from build123d import *

# Parameters (mm, degrees)
SKETCH_W        = 37.5
SKETCH_H        = 36
PAD_DEPTH       = 3.5
SKETCH001_R     = 1.05
POCKET_DEPTH    = 5
SKETCH002_R     = 1.6
POCKET001_DEPTH = 1.1
SKETCH003_W     = 10
SKETCH003_H     = 2.5
PAD001_DEPTH    = 5
SKETCH004_W     = 20
SKETCH004_H     = 2.5
PAD002_DEPTH    = 5
SKETCH005_W     = 7
SKETCH005_H     = 7
POCKET002_DEPTH = 5
FILLET_R        = 3
FILLET001_R     = 2


with BuildPart() as part:
    # Sketch → Pad (new body)
    with BuildSketch(Plane.XY):
        Rectangle(SKETCH_W, SKETCH_H)
    extrude(amount=PAD_DEPTH)

    # Sketch001 (on Face6 of Pad) → Pocket (cut)
    with BuildSketch(Plane.XY.offset(3.5)):
        with Locations((0, -14.25)):
            Circle(SKETCH001_R)
    extrude(amount=-POCKET_DEPTH, mode=Mode.SUBTRACT)

    # Sketch002 (on Face5 of Pocket) → Pocket001 (cut)
    with BuildSketch(Plane.XY.offset(3.5)):
        with Locations((0, -14.25)):
            Circle(SKETCH002_R)
    extrude(amount=-POCKET001_DEPTH, mode=Mode.SUBTRACT)

    # Sketch003 (on Face4 of Pocket001) → Pad001 (join)
    with BuildSketch(Plane(origin=(0, 0, 0), x_dir=(1, 0, 0), z_dir=(0, 0, -1))):
        with Locations((-10, 14.6)):
            Rectangle(SKETCH003_W, SKETCH003_H)
        with Locations((10, 14.6)):
            Rectangle(SKETCH003_W, SKETCH003_H)
    extrude(amount=PAD001_DEPTH)

    # Sketch004 (on Face4 of Pad001) → Pad002 (join)
    with BuildSketch(Plane(origin=(0, 0, 0), x_dir=(1, 0, 0), z_dir=(0, 0, -1))):
        with Locations((-4.75, -14.6)):
            Rectangle(SKETCH004_W, SKETCH004_H)
    extrude(amount=PAD002_DEPTH)

    # Sketch005 (on Face4 of Pad002) → Pocket002 (cut)
    with BuildSketch(Plane(origin=(0, 0, 0), x_dir=(1, 0, 0), z_dir=(0, 0, -1))):
        with Locations((15.25, -14.5)):
            Rectangle(SKETCH005_W, SKETCH005_H)
    extrude(amount=-POCKET002_DEPTH, mode=Mode.SUBTRACT)

    # Fillet
    fillet_edges = [part.edges().sort_by_distance(p)[0] for p in [
        (11.75, 11, 1.75),
    ]]
    fillet(fillet_edges, radius=FILLET_R)

    # Fillet001
    fillet001_edges = [part.edges().sort_by_distance(p)[0] for p in [
        (18.75, -18, 1.75),
        (-18.75, 18, 1.75),
        (-18.75, -18, 1.75),
    ]]
    fillet(fillet001_edges, radius=FILLET001_R)


solid = part.part
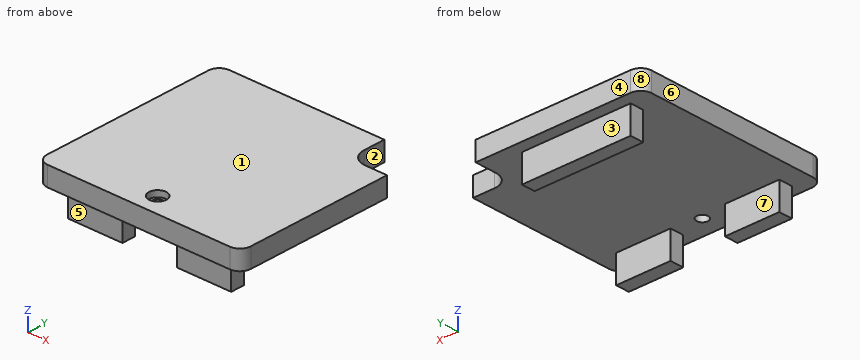
Verification items for the finished model (mm, model axes). Face numbers are marked on the shaded views. A direction names the side the tool comes from. Coordinates: 2 decimals unless noted, no trailing zeros. Order: outer loops, then holes, each group sorted by start corner. A loop starts at its lowest first (then second) coordinate and runs counter-clockwise, first axis right, second up. Notation, with made-up numbers: (11, 44.5) -> (33, 44.5) arc R20 ccw to (33, 48.5) -> close; hole circle Ø3 at (53.25, 31.25). An arc over 180 degrees is marked (long way). Put each result on its own line as item: value. Start each with the question number.
1. Cross-section at D-D, the plane z = 1.5. Record the boundary of the cut face in (x, y), then the cut area to 3 significant figures.
2. Cross-section at A-A, the plane x = 0. Record the boundary of the cut face in (y, z), then the cut area to 3 significant figures.
3. Mould release check, pull along Y, two halves, no side actions. Record for the marked faces 6, 7 and 8: released by +Y, released by -Y, zero draft, split by the parting line, or undercut.
4. Cross-section at C-C, the plane y = -14.25. Record the boundary of the cut face in (x, z), then the cut area to 3 significant figures.
5. Cross-section at B-B, the plane z = -3.75. Record the boundary of the cut face in (x, y).
6. Access from +Z, -Z, +X, -X, +Y, -Y to the whole of each face (thin tool, end or side, straight path). Record for the marked faces 1, 2, 3, 4 and 5.
7. Go/stop test with flat-tipped pins: pin 1 Ø1.2 at (y, z) = (14.5, -3.5) entering from -X; pin 2 Ø0.8 at (y, z) = (-15, -3) entering from +X; pin 3 Ø1 at (x, y) = (0, -14) entering from +Z; pin 4 Ø0.8 at (y, z) = (-15, -3.5) entering from -X. Record where each tip stops, or that it passes through.
8. Material ranges on L1, parallel to Y at x = -8, z = -4.25; L2, parallel to Y at x = 0, z = 3; L3, parallel to Z at x = 7.5, y = -3.5, recorded low to high. Write a range as [from, to].
Computed:
1. outline: (-18.75, -16) arc R2 ccw to (-16.75, -18) -> (16.75, -18) arc R2 ccw to (18.75, -16) -> (18.75, 11) -> (14.75, 11) arc R3 cw to (11.75, 14) -> (11.75, 18) -> (-16.75, 18) arc R2 ccw to (-18.75, 16) -> close; hole circle Ø2.1 at (0, -14.25)
1. area: 1,300 mm2
2. outline: (-18, 0) -> (-15.3, 0) -> (-15.3, 2.4) -> (-15.85, 2.4) -> (-15.85, 3.5) -> (-18, 3.5) -> close; (-13.2, 0) -> (13.35, 0) -> (13.35, -5) -> (15.85, -5) -> (15.85, 0) -> (18, 0) -> (18, 3.5) -> (-12.65, 3.5) -> (-12.65, 2.4) -> (-13.2, 2.4) -> close
2. area: 130 mm2
3. face 6: zero draft
3. face 7: undercut
3. face 8: released by +Y
4. outline: (-18.75, 0) -> (-15, 0) -> (-15, -5) -> (-5, -5) -> (-5, 0) -> (-1.05, 0) -> (-1.05, 2.4) -> (-1.6, 2.4) -> (-1.6, 3.5) -> (-18.75, 3.5) -> close; (1.05, 0) -> (5, 0) -> (5, -5) -> (15, -5) -> (15, 0) -> (18.75, 0) -> (18.75, 3.5) -> (1.6, 3.5) -> (1.6, 2.4) -> (1.05, 2.4) -> close
4. area: 223 mm2
5. outline: (-15, -15.85) -> (-5, -15.85) -> (-5, -13.35) -> (-15, -13.35) -> close; (-14.75, 13.35) -> (5.25, 13.35) -> (5.25, 15.85) -> (-14.75, 15.85) -> close; (5, -15.85) -> (15, -15.85) -> (15, -13.35) -> (5, -13.35) -> close
6. face 1: +Z, +X, -X, +Y, -Y
6. face 2: +Z, -Z, +X, +Y
6. face 3: -Z, +X, -X, +Y
6. face 4: +Z, -Z, +X, -X, +Y
6. face 5: -Z, +X, -X, -Y
7. pin 1: x = -14.75
7. pin 2: x = 15
7. pin 3: through
7. pin 4: x = -15
8. L1: [-15.85, -13.35], [13.35, 15.85]
8. L2: [-18, -15.85], [-12.65, 18]
8. L3: [0, 3.5]
